Check sheet for the modelled part. Datum: model origin and axes. Units: mm. Face numbers are marked on the shaded views. A direction names the side the tool comes from. Give positions to 0.01 mm unless a question says otherwise; leave off trailing zeros. Order: outer loops, then holes, each group sorted by start corner. A loop starts at its lowest first (then second) coordinate and runs counter-clockwise, first axis right, second up. Notation, with made-up numbers: M 68.25,70 L 108.25,70 A27 cw 108.25,94 Z; hole C -31.5,45 d2. An arc over 180 degrees is marked long. Return JSON: item names as keys, results as strings. Group by question number.
Autodesk Inventor part; units mm, degrees
ref_plane "YZ Plane" through (0, 0, 0) normal (1, 0, 0) x (0, 1, 0)
ref_plane "XZ Plane" through (0, 0, 0) normal (0, 1, 0) x (-1, 0, 0)
ref_plane "XY Plane" through (0, 0, 0) normal (0, 0, 1) x (1, 0, 0)
sketch "Sketch1" plane through (0, 0, 0) normal (0, 0, 1) x (1, 0, 0)
  line L0 (-93.9216, 0) -> (15.6536, 0)
  line L1 (0, -306.9874) -> (0, 252.5784)
  line L2 (0, 152.4) -> (0, -152.4)
  line L3 (0, 152.4) -> (-69.85, 31.4163)
  line L4 (0, -152.4) -> (-69.85, -31.4163)
  arc A0 (-69.85, 31.4163) -> (-69.85, -31.4163) centre (-15.4355, 0) ccw
  line L5 (-78.268, 172.6404) -> (-78.268, -227.0494) construction
  point P0 (0, 0)
  point P1 (0, 0)
  dimension "d0" = 304.8
  dimension "d13" = 30
  dimension "d14" = 139.7
extrude "Extrusion1" add sketch "Sketch1" along normal mid plane 609.6
sketch "Sketch3" plane through (0, 0, 0) normal (0, 1, 0) x (-1, 0, 0)
  line L0 (69.85, 304.8) -> (0, 304.8)
  line L1 (0, -304.8) -> (0, 304.8)
  line L2 (69.85, 304.8) -> (69.85, 304.8)
  line L3 (69.85, -304.8) -> (69.85, 304.8)
  line L4 (69.85, -304.8) -> (69.85, -304.8)
  line L5 (69.85, -304.8) -> (69.85, 304.8)
  line L6 (78.268, -304.8) -> (78.268, 304.8)
  line L7 (69.85, 304.8) -> (78.268, 304.8)
  line L8 (0, 304.8) -> (78.268, 259.612)
  point P0 (0, 0)
  dimension "d8" = 30
extrude "Extrusion3" cut sketch "Sketch3" along normal through all both and the other way through all
mirror "Mirror1" about plane through (0, 0, 0) normal (0, 0, 1) of "Extrusion3"
shell "Shell1" thickness 3.175 removed faces 1 at (0, -50.8, -101.6)
properties part number "front bumper"
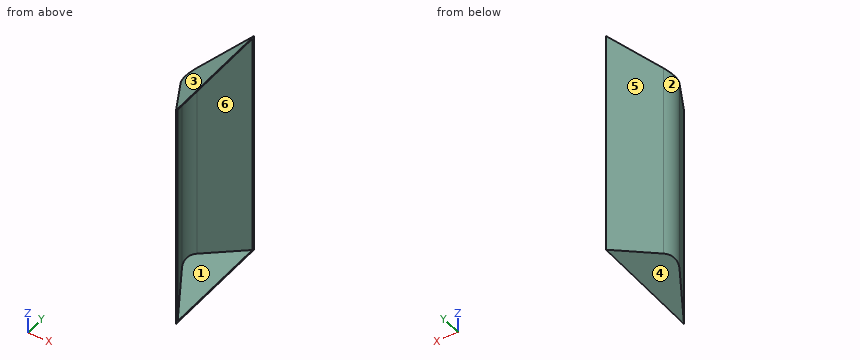
1) Sectioned sample at A-A on z = 25.5. Record the boundary of the cut face in (x, y).
2) Material ranges on line 1 along Y through (x, z) = (-57, -156.5); line 2 along Y through (x, z) = (-53, -180); line 3 along Z through (x, y) = (-10, -47), recorded low to high.
3) Release check for a two-part mould opening along Z. For the marked faces 1, 2, 3 and 4 record: released by +Z, released by -Z, zero draft, split by the parting line, or undercut.
4) Sectioned sample at B-B on x = -18.5. Record the boundary of the cut face in (y, z), then the cut area to 3 significant figures.
5) Depth check by flat-ended pin: P1, Ø3, axis at x = -33.5, z = -54, coming from the +Y side; P2, Ø10, axis at x = -52.5, z = 72, coming from the -Y side; P3, Ø4, axis at x = -24, z = -32.5, coming from the -Y side. Enter the tip coordinate at first touch or a pass-through.
6) Sectioned sample at C-C on y = -84.5. Record the boundary of the cut face in (x, z), then the cut area to 3 significant figures.
7) Tool access check on the marked faces 5 and 6. Record the directions out of +Z, -Z, +X, -X, +Y, -Y that give a thin tool (end or side, any length) a straight path to the whole face; none if there is none.
8) Sectioned sample at D-D on x = -52. Record the boundary of the cut face in (y, z), then the cut area to 3 significant figures.
Reply:
{
 "1": {"outline": "M -69.85,-31.42 L 0,-152.4 L 0,-146.05 L -67.1,-29.83 A59.66 cw -67.1,29.83 L 0,146.05 L 0,152.4 L -69.85,31.42 A62.83 ccw Z"},
 "2": {"line 1": "-53.67 to -47.32, 47.32 to 53.67", "line 2": "-60.6 to -54.25, 54.25 to 60.6", "line 3": "-299.03 to -295.36, 295.36 to 299.03"},
 "3": {"face 1": "undercut", "face 2": "zero draft", "face 3": "released by +Z", "face 4": "released by -Z"},
 "4": {"outline": "M -120.36,-294.12 L 120.36,-294.12 L 120.36,294.12 L -120.36,294.12 Z; hole M -114.01,-290.45 L 114.01,-290.45 L 114.01,290.45 L -114.01,290.45 Z", "area": "9,140 mm^2"},
 "5": {"P1": "y = 96.97", "P2": "y = -70.13", "P3": "y = -114.29"},
 "6": {"outline": "M -39.2,-282.17 L 0,-304.8 L 0,-301.13 L -35.54,-280.62 L -35.54,280.62 L 0,301.13 L 0,304.8 L -39.2,282.17 Z", "area": "2,340 mm^2"},
 "7": {"face 5": "+Z, -Z, -X, +Y", "face 6": "+X"},
 "8": {"outline": "M -62.33,-274.78 L 62.33,-274.78 L 62.33,274.78 L -62.33,274.78 Z; hole M -55.98,-271.11 L 55.98,-271.11 L 55.98,271.11 L -55.98,271.11 Z", "area": "7,800 mm^2"}
}
